```python
from build123d import *

# Parameters (mm, degrees)
F0_R          = 5.1
F1_DEPTH      = 45
F2_DEPTH      = 2.5
F6_START      = -5
F4_W          = 37
F4_H          = 38
F4_R          = 1.6
F4_R_2        = 12
F6_DEPTH      = 28
F7_DEPTH      = 5
F7_DEPTH_BACK = 16.5
F5_R          = 3
F8_DEPTH      = 16.5
F9_W          = 18
F9_H          = 10
F10_DEPTH     = 19.0834106782
F11_COUNT     = 3
F11_ANGLE     = 480


with BuildPart() as f1:
    # F0 (on Top) → F1 (new body)
    with BuildSketch(Plane.XY):
        with BuildLine():
            Line((48.3891499996, -27.9374887781), (0, 0))
            Line((0, 0), (-48.3891499996, -27.9374887781))
            ThreePointArc((-48.3891499996, -27.9374887781), (-37.0005953155, -59.5433683199), (-37.3249107961, -93.1369036932))
            ThreePointArc((-37.3249107961, -93.1369036932), (-26.5643472762, -85.0438685233), (-17.5, -95))
            ThreePointArc((-17.5, -95), (-20.2732115997, -101.9118397997), (-27.0547058834, -104.9900807379))
            Line((-27.0547058834, -104.9900807379), (27.4981817467, -104.9999998347))
            ThreePointArc((27.4981817467, -104.9999998347), (19.7989254456, -88.6208581527), (37.3249107961, -93.1369036932))
            ThreePointArc((37.3249107961, -93.1369036932), (37.0005953155, -59.5433683199), (48.3891499996, -27.9374887781))
        make_face()
        with BuildLine():
            ThreePointArc((37.5, -95), (37.4561314767, -94.0643472762), (37.3249107961, -93.1369036932))
            ThreePointArc((37.3249107961, -93.1369036932), (19.7989254456, -88.6208581527), (27.4981817467, -104.9999998347))
            ThreePointArc((27.4981817467, -104.9999998347), (34.570424933, -102.0717106323), (37.5, -95))
        make_face()
        with Locations((27.5, -95)):
            Circle(F0_R, mode=Mode.SUBTRACT)
        with BuildLine():
            ThreePointArc((-17.5, -95), (-26.5643472762, -85.0438685233), (-37.3249107961, -93.1369036932))
            ThreePointArc((-37.3249107961, -93.1369036932), (-35.342921879, -101.2039162148), (-27.9489269865, -104.9899181459))
            Line((-27.9489269865, -104.9899181459), (-27.0547058834, -104.9900807379))
            ThreePointArc((-27.0547058834, -104.9900807379), (-20.2732115997, -101.9118397997), (-17.5, -95))
        make_face()
        with Locations((-27.5, -95)):
            Circle(F0_R, mode=Mode.SUBTRACT)
    extrude(amount=F1_DEPTH)

    # F0 (on Top) → F2 (join)
    with BuildSketch(Plane.XY):
        with Locations((27.5, -95)):
            Circle(F0_R)
        with Locations((-27.5, -95)):
            Circle(F0_R)
    extrude(amount=F2_DEPTH)

    # F4 (on offset) → F6 (cut)
    with BuildSketch(Plane(origin=(-0.016090632, -88.4949967703, 0), x_dir=(0.9999999835, -0.0001818253, 0), z_dir=(-0.0001818253, -0.9999999835, 0)).offset(F6_START)):
        with Locations((0, 19)):
            Rectangle(F4_W, F4_H)
        with Locations((-13, 6)):
            Circle(F4_R, mode=Mode.SUBTRACT)
        with Locations((13, 6)):
            Circle(F4_R, mode=Mode.SUBTRACT)
        with Locations((-13, 32)):
            Circle(F4_R, mode=Mode.SUBTRACT)
        with Locations((0, 19)):
            Circle(F4_R_2, mode=Mode.SUBTRACT)
        with Locations((13, 32)):
            Circle(F4_R, mode=Mode.SUBTRACT)
        with Locations((0, 19)):
            Circle(F4_R_2)
        with Locations((-13, 32)):
            Circle(F4_R)
        with Locations((13, 32)):
            Circle(F4_R)
        with Locations((13, 6)):
            Circle(F4_R)
        with Locations((-13, 6)):
            Circle(F4_R)
    extrude(amount=-F6_DEPTH, mode=Mode.SUBTRACT)

    # F4 (on offset) → F7 (cut, two sides)
    with BuildSketch(Plane(origin=(-0.016090632, -88.4949967703, 0), x_dir=(0.9999999835, -0.0001818253, 0), z_dir=(-0.0001818253, -0.9999999835, 0))) as f7_sk:
        with Locations((0, 19)):
            Circle(F4_R_2)
        with Locations((-13, 32)):
            Circle(F4_R)
        with Locations((13, 32)):
            Circle(F4_R)
        with Locations((-13, 6)):
            Circle(F4_R)
        with Locations((13, 6)):
            Circle(F4_R)
    extrude(amount=-F7_DEPTH, mode=Mode.SUBTRACT)
    extrude(f7_sk.sketch, amount=F7_DEPTH_BACK, mode=Mode.SUBTRACT)

    # F5 (on face) → F8 (cut)
    with BuildSketch(Plane(origin=(-0.0190907499, -104.9949964975, 0), x_dir=(0.9999999835, -0.0001818253, 0), z_dir=(-0.0001818253, -0.9999999835, 0))):
        with Locations((-13, 32)):
            Circle(F5_R)
        with Locations((13, 32)):
            Circle(F5_R)
        with Locations((13, 6)):
            Circle(F5_R)
        with Locations((-13, 6)):
            Circle(F5_R)
    extrude(amount=-F8_DEPTH, mode=Mode.SUBTRACT)

    # F9 (on face) → F10 (cut, up to face)
    with BuildSketch(Plane.XY.offset(45)):
        Polygon((9, -83.4966360413), (-9, -83.4933631854), (-9, -90), (9, -90), align=None)
        with Locations((0, -95)):
            Rectangle(F9_W, F9_H)
    extrude(amount=-F10_DEPTH, mode=Mode.SUBTRACT)

    # F11: F1 ×3 about axis
    f11_axis = Axis((0, 0, 0), (0, 0, 1))


with BuildPart() as f1_1:
    add(f1.part)
    for i in range(1, F11_COUNT):
        add(f1.part.rotate(f11_axis, i * F11_ANGLE / (F11_COUNT - 1)))


solid = f1_1.part
```
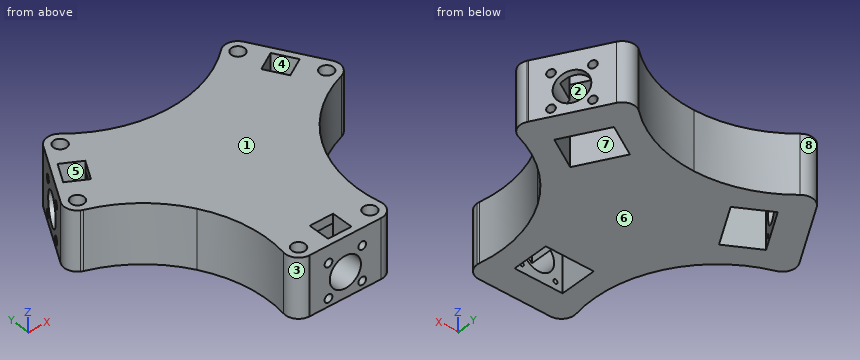
The listing builds one solid part. Answer for the finished solid, in the listing's coordinates (mm). Face numbers are marked on the shaded views. A direction names the side the tool comes from. Round coordinates to 2 decimals unless told otherwise and drop trailing zeros. Write each loop counter-clockwise with the first axis right and the second up, starting at its lowest first coordinate (ties: lowest second). Pieces come first, ordered by that corner, then holes. Notation, with made-up numbers: (-30, 29) -> (-17, 29) arc R28 ccw to (-17, 62) -> close; hole circle Ø8 at (80, 19.25). An arc over 180 degrees is marked (long way). Answer as a JSON object with one key per item and string values. Group by question number.
Q1. Determine the mould class of the marked faces 1, 2, 3 and 4 for opening direction X: pulls with the +X half, pulls with the -X half, needs draft (parallel to the pull), parting line crosses it, or undercut.
Q2. Each of these flat-tipped pins is pushed along its axis until it touches: pin 1 Ø2 at (x, y) = (-15, -75.5) entering from -Z; pin 2 Ø3 at (x, z) = (-14, 30.5) entering from -Y; pin 3 Ø1 at (y, z) = (22, 18) entering from +X. Where does it stop, or does it pass through?
Q3. Section A-A (x = -6) is taken. Count the separate pieces of the cut face and the enclosed holes in it, plus the area to 3 significant figures.
Q4. Section C-C (y = -48) is taken. Write down the section's boundary in (x, z).
Q5. Straight lines are drawn through the part: line 1 along Z through (x, y) = (90, 36.5); line 2 along X through (y, z) = (-76, 27.5); line 3 along Y through (x, z) = (-70.5, 43). For each, find the intervals that lie inside material, in ascending order.
Q6. Which of the six approach directions +Z, -Z, +X, -X, +Y, -Y give full straight-line access (tool end or side, diameter ignored) to the marked faces 5, 6, 7 and 8?
Check values:
{
 "1": {"face 1": "needs draft", "face 2": "undercut", "face 3": "pulls with the -X half", "face 4": "undercut"},
 "2": {"pin 1": "z = 38", "pin 2": "y = -104.99", "pin 3": "x = 105.95"},
 "3": {"separate pieces": "3", "enclosed holes": "0", "area": "5,480 mm^2"},
 "4": {"outline": "(-39.71, 0) -> (39.71, 0) -> (39.71, 45) -> (-39.71, 45) -> close"},
 "5": {"line 1": "0 to 3.02, 8.98 to 29.02, 34.98 to 45", "line 2": "-35.66 to -18.51, 18.49 to 35.66", "line 3": "-1.91 to 44.88, 51.1 to 66.61, 76.02 to 81.12"},
 "6": {"face 5": "+Z", "face 6": "-Z, +X, -X, +Y, -Y", "face 7": "-Z", "face 8": "+Z, -Z, +Y"}
}
